Here's how the part is built. I have some questions about the finished solid (model axes, mm). A direction names the side the tool comes from. Round coordinates to 2 decimals unless told otherwise and drop trailing zeros. Order: outer loops, then holes, each group sorted by start corner. A loop starts at its lowest first (then second) coordinate and runs counter-clockwise, first axis right, second up. Notation, with made-up numbers: (61, 48.5) -> (95, 48.5) arc R20 cw to (95, 83.5) -> close; hole circle Ø6 at (71.5, 17.25). An arc over 180 degrees is marked (long way). One line per item, written item: value.
```python
from build123d import *

# Parameters (mm, degrees)
SKETCH_1_R          = 1.5
SKETCH_1_R_2        = 2
SKETCH_1_R_3        = 1.65
EXTRUDE_1_DEPTH     = 3
SKETCH_3_R          = 1
CUT_EXTRUDE_3_DEPTH = 124.273070863
SKETCH_4_R          = 24
SKETCH_4_R_2        = 13.5
SKETCH_4_R_3        = 7.5
CUT_EXTRUDE_4_DEPTH = 124.273070863
SKETCH_5_W          = 6
SKETCH_5_H          = 16.5
EXTRUDE_1_2_DEPTH   = 3
FILLET_4_R          = 1
FILLET_6_R          = 5
FILLET_7_R          = 3


with BuildPart() as part:
    # Sketch 1 → Extrude 1 (new body)
    with BuildSketch(Plane(origin=(0, 0, 0), x_dir=(1, 0, 0), z_dir=(0, 1, 0))):
        with BuildLine():
            Line((-51.003122908, 26.550545261), (-40.35899291, 21.009561902))
            ThreePointArc((-40.35899291, 21.009561902), (0, -45.5), (40.35899291, 21.009561902))
            Line((40.35899291, 21.009561902), (51.003122908, 26.550545261))
            ThreePointArc((51.003122908, 26.550545261), (57.123657521, 6.567933576), (55.697982668, -14.282322175))
            Line((55.697982668, -14.282322175), (35, -95))
            Line((35, -95), (35, -105))
            Line((35, -105), (20, -105))
            Line((20, -105), (20, -109))
            Line((20, -109), (-20, -109))
            Line((-20, -109), (-20, -105))
            Line((-20, -105), (-35, -105))
            Line((-35, -105), (-35, -95))
            Line((-35, -95), (-55.697982668, -14.282322175))
            ThreePointArc((-55.697982668, -14.282322175), (-57.123657521, 6.567933576), (-51.003122908, 26.550545261))
        make_face()
        with Locations(Location((-31, -100, 0), (0, 0, 270))):
            Circle(SKETCH_1_R, mode=Mode.SUBTRACT)
        with Locations(Location((31, -100, 0), (0, 0, 90))):
            Circle(SKETCH_1_R, mode=Mode.SUBTRACT)
        with Locations(Location((-37.123106012, -37.123106012, 0), (0, 0, 270))):
            Circle(SKETCH_1_R_2, mode=Mode.SUBTRACT)
        with Locations(Location((-52.5, 0, 0), (0, 0, 270))):
            Circle(SKETCH_1_R_2, mode=Mode.SUBTRACT)
        with Locations(Location((52.5, 0, 0), (0, 0, 270))):
            Circle(SKETCH_1_R_2, mode=Mode.SUBTRACT)
        with Locations(Location((37.123106012, -37.123106012, 0), (0, 0, 270))):
            Circle(SKETCH_1_R_2, mode=Mode.SUBTRACT)
        with Locations(Location((32.925309654, -89, 0), (0, 0, 270))):
            Circle(SKETCH_1_R_3, mode=Mode.SUBTRACT)
        with Locations(Location((36.65113283, -74.470091478, 0), (0, 0, 270))):
            Circle(SKETCH_1_R_3, mode=Mode.SUBTRACT)
    extrude(amount=EXTRUDE_1_DEPTH)

    # Sketch 3 → Cut-Extrude 3 (cut, through all)
    with BuildSketch(Plane(origin=(0, 3, 0), x_dir=(1, 0, 0), z_dir=(0, 1, 0))):
        with Locations((-21, -105)):
            Circle(SKETCH_3_R)
        with Locations((21, -105)):
            Circle(SKETCH_3_R)
    extrude(amount=-CUT_EXTRUDE_3_DEPTH, mode=Mode.SUBTRACT)

    # Sketch 4 → Cut-Extrude 4 (cut, through all)
    # profile 1 of 4: a face of its own
    with BuildSketch(Plane(origin=(0, 3, 0), x_dir=(1, 0, 0), z_dir=(0, 1, 0))):
        with Locations(Location((0, -76, 0), (0, 0, 270))):
            Circle(SKETCH_4_R)
        with Locations(Location((0, -76, 0), (0, 0, 270))):
            Circle(SKETCH_4_R_2, mode=Mode.SUBTRACT)
    # profile 2 of 4: a face of its own
    with BuildSketch(Plane(origin=(0, 3, 0), x_dir=(1, 0, 0), z_dir=(0, 1, 0))):
        with Locations(Location((0, -76, 0), (0, 0, 270))):
            Circle(SKETCH_4_R_3)
    # profile 3 of 4: a face of its own
    with BuildSketch(Plane(origin=(0, 3, 0), x_dir=(1, 0, 0), z_dir=(0, 1, 0))):
        with BuildLine():
            Line((-35.830489881, -51.50170866), (-31.190656418, -69.59606059))
            ThreePointArc((-31.190656418, -69.59606059), (-29.717442346, -70.72334194), (-28.275157423, -69.556749833))
            ThreePointArc((-28.275157423, -69.556749833), (-24.920071276, -61.167938525), (-19.146204544, -54.21875))
            ThreePointArc((-19.146204544, -54.21875), (-25.395621297, -51.58790962), (-31.291887936, -48.239690602))
            ThreePointArc((-31.291887936, -48.239690602), (-34.67538019, -48.320471942), (-35.830489881, -51.50170866))
        make_face()
    # profile 4 of 4: a face of its own
    with BuildSketch(Plane(origin=(0, 3, 0), x_dir=(1, 0, 0), z_dir=(0, 1, 0))):
        with BuildLine():
            Line((35.830489881, -51.50170866), (31.190656418, -69.59606059))
            ThreePointArc((31.190656418, -69.59606059), (29.717442346, -70.72334194), (28.275157423, -69.556749833))
            ThreePointArc((28.275157423, -69.556749833), (24.920071276, -61.167938525), (19.146204544, -54.21875))
            ThreePointArc((19.146204544, -54.21875), (25.395621297, -51.58790962), (31.291887936, -48.239690602))
            ThreePointArc((31.291887936, -48.239690602), (34.67538019, -48.320471942), (35.830489881, -51.50170866))
        make_face()
    extrude(amount=-CUT_EXTRUDE_4_DEPTH, mode=Mode.SUBTRACT)


with BuildPart() as cut_extrude_4_piece_1:
    # of the separate pieces the step leaves, piece 1, a body of its own (cut_extrude_4_pieces)
    add(part.part.solids().sort_by_distance((-51.003122908, 0, -26.550545261))[0])



with BuildPart() as cut_extrude_4_piece_2:
    # of the separate pieces the step leaves, piece 2, a body of its own (cut_extrude_4_pieces)
    add(part.part.solids().sort_by_distance((0, 0, 89.5))[0])


with BuildPart() as cut_extrude_4_piece_1_1:
    add(cut_extrude_4_piece_1.part)

    add(cut_extrude_4_piece_2.part)  # Extrude 1 2 merges Cut-Extrude 4 piece 2
    # Sketch 5 → Extrude 1 2 (add)
    with BuildSketch(Plane(origin=(0, 3, 0), x_dir=(1, 0, 0), z_dir=(0, 1, 0))):
        with Locations((0, -60.25)):
            Rectangle(SKETCH_5_W, SKETCH_5_H)
        Polygon((22.284609691, -85.401923789), (7.995190528, -77.151923789), (4.995190528, -82.348076211), (19.284609691, -90.598076211), align=None)
        Polygon((-19.284609691, -90.598076211), (-4.995190528, -82.348076211), (-7.995190528, -77.151923789), (-22.284609691, -85.401923789), align=None)
    extrude(amount=-EXTRUDE_1_2_DEPTH)

    # Fillet 4
    fillet_4_edges = [cut_extrude_4_piece_1_1.edges().sort_by_distance(p)[0] for p in [
        (19.121590627, 1.5, 90.503957111),
        (22.121590627, 1.5, 85.307804688),
        (-19.146204544, 1.5, 54.21875),
        (19.146204544, 1.5, 54.21875),
        (-22.121590627, 1.5, 85.307804688),
        (-19.121590627, 1.5, 90.503957111),
        (3, 1.5, 52.1882382),
        (-3, 1.5, 52.1882382),
        (-35, 1.5, 105),
        (-20, 1.5, 109),
        (20, 1.5, 109),
        (35, 1.5, 105),
    ]]
    fillet(fillet_4_edges, radius=FILLET_4_R)

    # Fillet 6
    fillet_6_edges = [cut_extrude_4_piece_1_1.edges().sort_by_distance(p)[0] for p in [
        (-35, 1.5, 95),
        (35, 1.5, 95),
    ]]
    fillet(fillet_6_edges, radius=FILLET_6_R)

    # Fillet 7
    fillet_7_edges = [cut_extrude_4_piece_1_1.edges().sort_by_distance(p)[0] for p in [
        (9.899013115, 1.5, 85.179299502),
        (12.899013115, 1.5, 79.983147079),
        (-9.899013115, 1.5, 85.179299502),
        (-12.899013115, 1.5, 79.983147079),
        (51.003122908, 1.5, -26.550545261),
        (3, 1.5, 62.837553419),
        (40.35899291, 1.5, -21.009561902),
        (-40.35899291, 1.5, -21.009561902),
        (-3, 1.5, 62.837553419),
        (-51.003122908, 1.5, -26.550545261),
    ]]
    fillet(fillet_7_edges, radius=FILLET_7_R)


solid = cut_extrude_4_piece_1_1.part
```
Q1. I want a section at A-A on x = 0. Write out the boundary of the cut face in (y, z).
Answers:
outline: (0, 45.5) -> (3, 45.5) -> (3, 68.5) -> (0, 68.5) -> close; (0, 83.5) -> (3, 83.5) -> (3, 89.5) -> (0, 89.5) -> close; (0, 100) -> (3, 100) -> (3, 109) -> (0, 109) -> close
Q2. If we mould it in two halves opening along Z, with no side actions, what happens to faces 1 (the face through (57.26, 1.48, -5.26)), 2 (the face through (-29.735, 1.479, 100.806)), 3 (the face through (-25.376, 1.521, 61.962)), 4 (the face through (-45.284, 1.479, 54.896))? For each: pulls with the +Z half, pulls with the -Z half, needs draft (parallel to the pull), parting line crosses it, or undercut.
Answers:
face 1: parting line crosses it
face 2: undercut
face 3: undercut
face 4: pulls with the +Z half
Q3. Which directions (+Z, -Z, +X, -X, +Y, -Y) give clear straight access to the entire face, cutting with the end or side of a thin tool? Please do faces 5 (the face through (-45.64, 1.48, -23.76)), 6 (the face through (-15.01, 1.52, 88.13)).
Answers:
face 5: -Z, +Y, -Y
face 6: +Y, -Y
Q4. I want a section at C-C on x = 26. Write out the boundary of the cut face in (y, z), then the cut area to 3 significant figures.
Answers:
outline: (0, 37.34) -> (3, 37.34) -> (3, 51.29) -> (0, 51.29) -> close; (0, 63.15) -> (3, 63.15) -> (3, 105) -> (0, 105) -> close
area: 167 mm2
Q5. For P1, Ø5, axis at x = 37.12, z = 37.12, coming from the -Y side; P2, Ø0.9, axis at y = 1, z = 98.5, coming from the -X side; P3, Ø3, axis at x = -52.5, z = 0, coming from the -Y side; P4, Ø0.9, axis at y = 1.5, z = 106, coming from the -X side, each with a flat end and sliding along its axis, tell me the tip position at first contact or that it passes through.
Answers:
P1: y = 0
P2: x = -35
P3: through
P4: x = -20
Q6. I want a section at B-B on z = 0. Write out the boundary of the cut face in (x, y).
Answers:
outline: (-57.5, 0) -> (-54.5, 0) -> (-54.5, 3) -> (-57.5, 3) -> close; (-50.5, 0) -> (-45.5, 0) -> (-45.5, 3) -> (-50.5, 3) -> close; (45.5, 0) -> (50.5, 0) -> (50.5, 3) -> (45.5, 3) -> close; (54.5, 0) -> (57.5, 0) -> (57.5, 3) -> (54.5, 3) -> close
Q7. I want a section at D-D on z = 43.5. Write out the boundary of the cut face in (x, y).
Answers:
outline: (-48.21, 0) -> (-13.34, 0) -> (-13.34, 3) -> (-48.21, 3) -> close; (13.34, 0) -> (48.21, 0) -> (48.21, 3) -> (13.34, 3) -> close
Q8. I need wall thicknesses on line 1 along X through (y, z) = (2.3, 0); line 2 along Z through (x, y) = (-16, 2.7); line 3 along Z through (x, y) = (-20.5, 0.95). Which ranges of each line are inside material? Lowest first, please.
Answers:
line 1: -57.5 to -54.5, -50.5 to -45.5, 45.5 to 50.5, 54.5 to 57.5
line 2: 42.59 to 58.11, 81.77 to 88.7, 93.89 to 109
line 3: 40.62 to 53.74, 55.49 to 63.52, 84.37 to 104.13
